The listing builds one solid part. Answer for the finished solid, in the listing's coordinates (mm). Face numbers are marked on the shaded views. A direction names the side the tool comes from. Round coordinates to 2 decimals unless told otherwise and drop trailing zeros. Write each loop counter-clockwise with the first axis right and the second up, starting at its lowest first coordinate (ties: lowest second). Pieces come first, ordered by that corner, then holes.
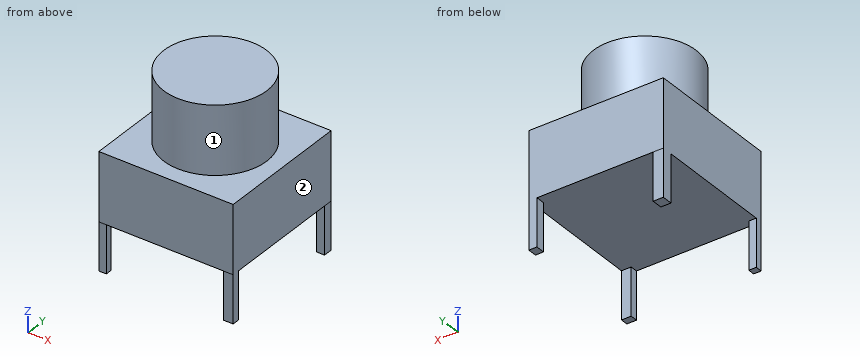
from build123d import *

# Parameters (mm, degrees)
F0_R     = 57.97101
F1_DEPTH = 76.556459
F3_DEPTH = 76.509021
F4_W     = 11.437774
F4_H     = 11.928283
F4_W_2   = 9.122617
F4_H_2   = 10.233626
F4_W_3   = 10.927506
F4_H_3   = 8.273392
F4_W_4   = 8.41286
F4_H_4   = 7.608004
F5_DEPTH = 53.518422


with BuildPart() as f1:
    # F0 (on Top) → F1 (new body)
    with BuildSketch(Plane.XY):
        Circle(F0_R)
    extrude(amount=F1_DEPTH)

    # F2 (on Top) → F3 (join)
    with BuildSketch(Plane.XY):
        Polygon((-75.723298, -76.582767), (75.636029, -76.763391), (75.636029, 75.860277), (-75.723298, 75.860277), align=None)
    extrude(amount=-F3_DEPTH)

    # F4 (on face) → F5 (join)
    with BuildSketch(Plane(origin=(0, 0, -76.509021), x_dir=(1, 0, 0), z_dir=(0, 0, -1))):
        with Locations((-70.004411, -69.896135)):
            Rectangle(F4_W, F4_H)
        with Locations((71.07472, -70.743464)):
            Rectangle(F4_W_2, F4_H_2)
        with Locations((70.172276, 72.626695)):
            Rectangle(F4_W_3, F4_H_3)
        with Locations((-71.516868, 72.778765)):
            Rectangle(F4_W_4, F4_H_4)
    extrude(amount=F5_DEPTH)


solid = f1.part
1. Section A-A on z = -82 is taken. Determine the outline of the cut face in (x, y).
Geometry says:
outline: (-75.72, -76.58) - (-67.31, -76.58) - (-67.31, -68.97) - (-75.72, -68.97) - close; (-75.72, 63.93) - (-64.29, 63.93) - (-64.29, 75.86) - (-75.72, 75.86) - close; (64.71, -76.76) - (75.64, -76.76) - (75.64, -68.49) - (64.71, -68.49) - close; (66.51, 65.63) - (75.64, 65.63) - (75.64, 75.86) - (66.51, 75.86) - close
2. Section D-D on z = 28.5 is taken. Determine the outline of the cut face in (x, y).
Geometry says:
outline: circle Ø115.94 at (0, 0)
3. Section C-C on x = 53.5 is taken. Determine the outline of the cut face in (y, z), plus the area to 3 significant figures.
Geometry says:
outline: (-76.74, -76.51) - (75.86, -76.51) - (75.86, 0) - (22.32, 0) - (22.32, 76.56) - (-22.32, 76.56) - (-22.32, 0) - (-76.74, 0) - close
area: 15,100 mm2
4. A tool of negligible diameter and unlimited length cuts with its end or side. For the marked faces 1 and 2, from which of +Z, -Z, +X, -X, +Y, -Y can it reach the whole face along a straight path? Write none if from no direction.
Geometry says:
face 1: +Z
face 2: +Z, -Z, +X, +Y, -Y
5. Section B-B on y = 0 is taken. Determine the outline of the cut face in (x, z).
Geometry says:
outline: (-75.72, -76.51) - (75.64, -76.51) - (75.64, 0) - (57.97, 0) - (57.97, 76.56) - (-57.97, 76.56) - (-57.97, 0) - (-75.72, 0) - close
6. Straight lines are drawn through the part: line 1 along X through (y, z) = (69.5, -103.5); line 2 along Z through (x, y) = (-41.5, 33); line 3 along Z through (x, y) = (68.5, 28.5). For each, find the intervals that lie inside material, in ascending order.
Geometry says:
line 1: x = -75.72 to -64.29, 66.51 to 75.64
line 2: z = -76.51 to 76.56
line 3: z = -76.51 to 0
7. Given pin 1 (5 mm diameter, centred on x = -16, z = 23, fed in from +Y); pin 2 (3 mm diameter, centred on x = 35, z = -77.5, fed in from -Y); pin 3 (5 mm diameter, centred on x = -53.5, z = -53, fed in from -Y), each flat-ended and moving along its own axis, determine where each tip first touches the part or whether it passes through.
Geometry says:
pin 1: stops at y = 56.38
pin 2: stops at y = -76.72
pin 3: stops at y = -76.61
